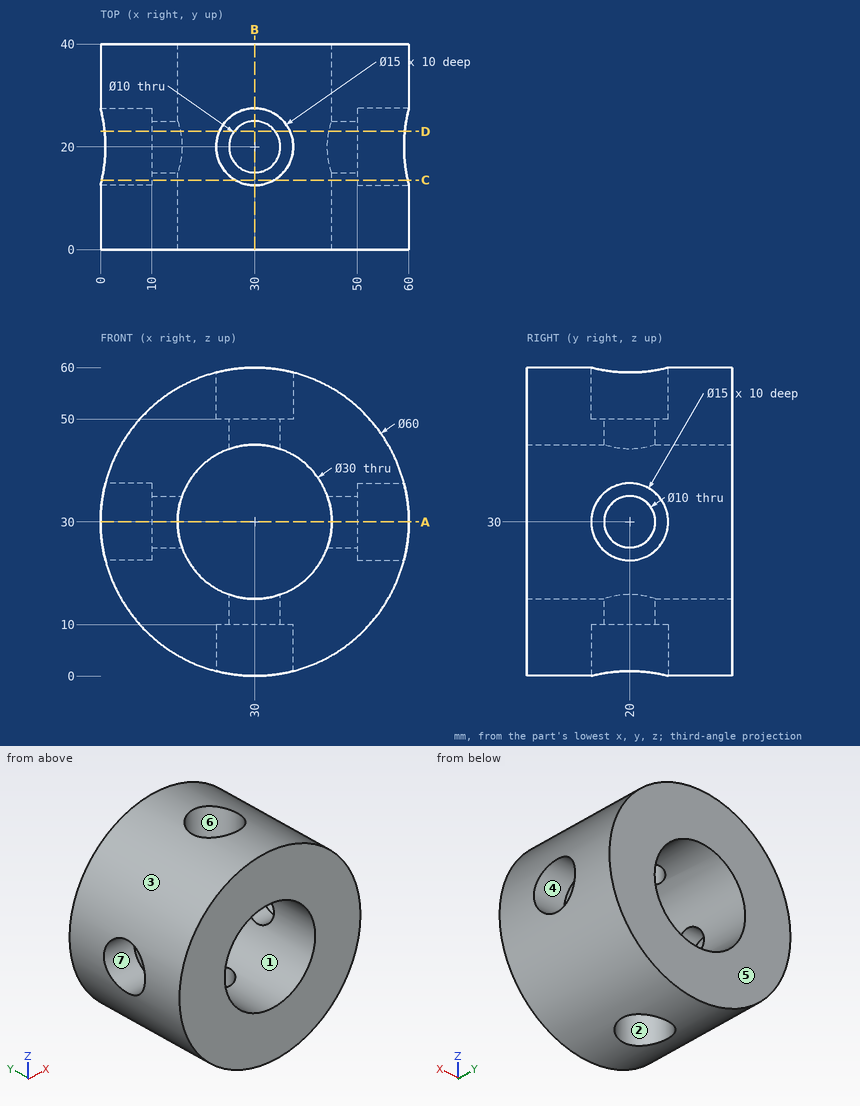
Geometry: see drawing. Coordinates: mm, zero at the bounding-box minimum. A direction names the side the tool comes from. Give positions to 0.01 mm unless a question says otherwise; leave off trailing zeros. Loops run counter-clockwise (first coordinate to the right, second up) from the corner with the lowest first, then second, coordinate; pieces in that order, holes last. Notation, with made-up numbers: (78, 38) - (121, 38) arc R34 ccw to (121, 71) - close; hole circle Ø8 at (10.5, 48). An arc over 180 degrees is marked (long way). Use CSV: the item, a comma, the result in double quotes. Start each with the question number.
Item 1: Section A-A on z = 30. Return loops of the section in (x, y).
Item 2: Line query: line 1 (Z direction, x = 30.5, y = 2); line 2 (Y direction, x = 30, z = 47.95); line 3 (Y direction, x = 30, z = 7). Output: solid intervals per line, ascending.
Item 3: Section C-C on y = 13.5. Return loops of the section in (x, z).
Item 4: Section B-B on x = 30. Return loops of the section in (y, z), then the cut area to 3 significant figures.
Item 5: Mould query, pull axis Z, two halves, no side actions, for the marked faces 1, 2, 3 and 4. Classes: pulls with the +Z half, pulls with the -Z half, needs draft (parallel to the pull), parting line crosses it, or undercut.
Item 6: Contact query for flat-ended pins moving along their axis: P1, Ø3, axis at x = 14.5, y = 24, coming from the -Z side; P2, Ø12, axis at x = 31, y = 17, coming from the +Z side; P3, Ø1, axis at y = 12, z = 26, coming from the -X side; P4, Ø13, axis at y = 20, z = 30, coming from the -X side. Output: stop coordinate, or through.
Item 7: Reachability of the marked faces 5, 6 and 7 from +Z, -Z, +X, -X, +Y, -Y: full face, straight path, thin tool, end or side. Return the list, or none.
Item 8: Section D-D on y = 23. State how many separate pieces and enclosed holes the cut face has, then the cut area to 3 significant figures.
Ans:
1,outline,"(0, 0) - (15, 0) - (15, 15) - (10, 15) - (10, 12.5) - (0, 12.5) - close; (0, 27.5) - (10, 27.5) - (10, 25) - (15, 25) - (15, 40) - (0, 40) - close; (45, 0) - (60, 0) - (60, 12.5) - (50, 12.5) - (50, 15) - (45, 15) - close; (45, 25) - (50, 25) - (50, 27.5) - (60, 27.5) - (60, 40) - (45, 40) - close"
2,line 1,"z = 0 to 15.01, 44.99 to 60"
2,line 2,"y = 0 to 15, 25 to 40"
2,line 3,"y = 0 to 12.5, 27.5 to 40"
3,outline,"(0.23, 26.26) arc R30 ccw to (26.26, 0.23) - (26.26, 10) - (33.74, 10) - (33.74, 0.23) arc R30 ccw to (59.77, 26.26) - (50, 26.26) - (50, 33.74) - (59.77, 33.74) arc R30 ccw to (33.74, 59.77) - (33.74, 50) - (26.26, 50) - (26.26, 59.77) arc R30 ccw to (0.23, 33.74) - (10, 33.74) - (10, 26.26) - close; hole circle Ø30 at (30, 30)"
4,outline,"(0, 0) - (12.5, 0) - (12.5, 10) - (15, 10) - (15, 15) - (0, 15) - close; (0, 45) - (15, 45) - (15, 50) - (12.5, 50) - (12.5, 60) - (0, 60) - close; (25, 10) - (27.5, 10) - (27.5, 0) - (40, 0) - (40, 15) - (25, 15) - close; (25, 45) - (40, 45) - (40, 60) - (27.5, 60) - (27.5, 50) - (25, 50) - close"
4,area,"800 mm2"
5,face 1,"undercut"
5,face 2,"needs draft"
5,face 3,"parting line crosses it"
5,face 4,"undercut"
6,P1,"stops at z = 3.47"
6,P2,"stops at z = 60"
6,P3,"stops at x = 0.2"
6,P4,"stops at x = 10"
7,face 5,"+Z, -Z, +X, -X, +Y"
7,face 6,"+Z"
7,face 7,"-X"
8,separate pieces,"4"
8,enclosed holes,"0"
8,area,"1,420 mm2"
